Here's the drawing with two shaded views (mm, measured from the low corner). I have some questions. Coordinates: 2 decimals unless noted, no trailing zeros. Write each loop counter-clockwise with the first axis right and the second up, starting at its lowest first coordinate (ties: lowest second). Pieces come first, ordered by that corner, then holes. Notation, with made-up numbers: (-39, 62) -> (-25, 62) arc R26 ccw to (-25, 98) -> close; hole circle Ø3 at (6, -34). An arc over 180 degrees is marked (long way). Put each result on its own line as item: value.
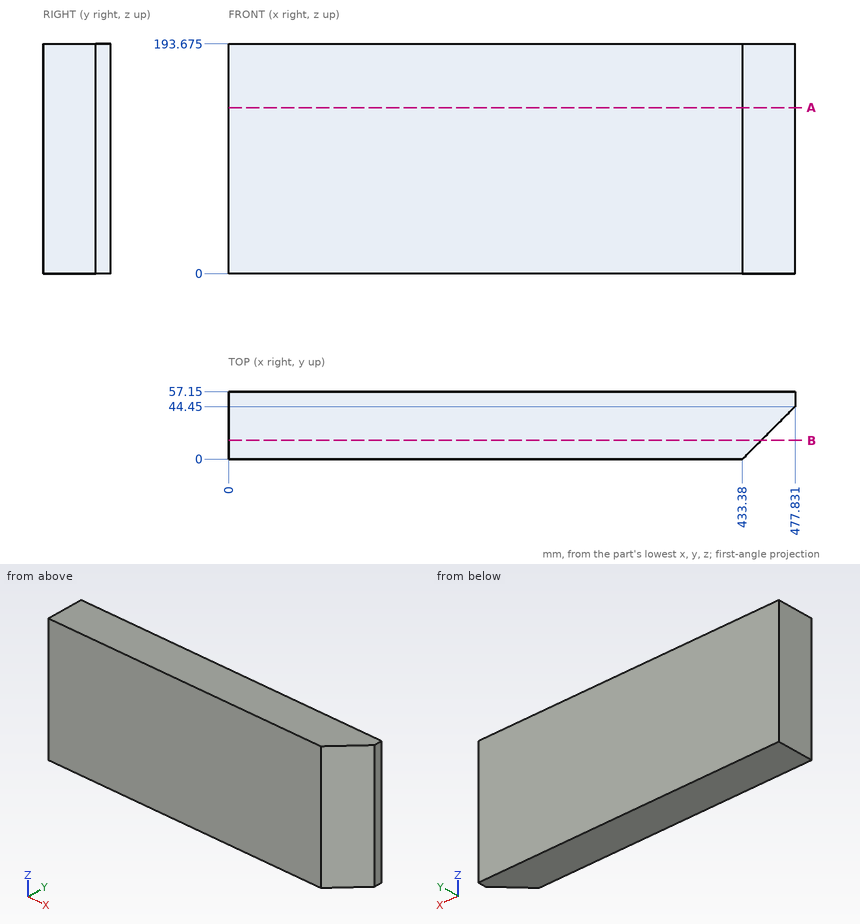
Item 1: Please list where these lines run through material, in increasing order: line 1 along X through (y, z) = (12, 26); line 2 along X through (y, z) = (4.5, 25); line 3 along Y through (x, z) = (449, 178). Write a range as from..to.
Output:
line 1: x = 0..445.38
line 2: x = 0..437.88
line 3: y = 15.62..57.15
Item 2: Imagine slicing it at B-B on y = 16. Write out the boundary of the cut face in (x, z) (1 decimal).
Output:
outline: (0, 0) -> (449.4, 0) -> (449.4, 193.7) -> (0, 193.7) -> close
Item 3: Imagine slicing it at A-A on z = 140. Write out the boundary of the cut face in (x, y), then the cut area to 3 significant figures.
Output:
outline: (0, 0) -> (433.38, 0) -> (477.83, 44.45) -> (477.83, 57.15) -> (0, 57.15) -> close
area: 26,300 mm²
